Autodesk Inventor part; units mm, degrees
ref_plane "YZ Plane" through (0, 0, 0) normal (1, 0, 0) x (0, 1, 0)
ref_plane "XZ Plane" through (0, 0, 0) normal (0, 1, 0) x (-1, 0, 0)
ref_plane "XY Plane" through (0, 0, 0) normal (0, 0, 1) x (1, 0, 0)
sketch "Sketch1" plane through (0, 0, 0) normal (0, 1, 0) x (-1, 0, 0)
  line L0 (0, 0) -> (464.159, 0) construction
  line L1 (464.159, 0) -> (464.159, -207.7664) construction
  line L2 (464.159, -207.7664) -> (0, -207.7664) construction
  line L3 (0, -207.7664) -> (0, 0) construction
  line L4 (89.199, -168.5726) -> (89.199, -173.9719)
  line L5 (89.199, -173.9719) -> (86.6636, -173.9719)
  line L6 (86.6636, -173.9719) -> (86.6636, -176.4581)
  line L7 (86.6636, -176.4581) -> (71.2328, -176.4581)
  line L8 (71.2328, -176.4581) -> (71.2328, -186.2934)
  line L9 (71.2328, -186.2934) -> (90.3359, -186.2934)
  line L10 (90.3359, -186.2934) -> (90.3359, -179.7626)
  line L11 (90.3359, -179.7626) -> (92.1613, -179.7626)
  line L12 (92.1613, -179.7626) -> (92.1613, -177.2606)
  line L13 (92.1613, -177.2606) -> (99.2738, -177.2606)
  line L14 (99.2738, -177.2606) -> (99.2738, -159.6681)
  line L15 (99.2738, -159.6681) -> (106.4808, -159.6681)
  line L16 (106.4808, -159.6681) -> (106.4808, -177.355)
  line L17 (106.4808, -177.355) -> (116.4572, -177.355)
  line L18 (116.4572, -177.355) -> (116.4572, -149.6917)
  line L19 (116.4572, -149.6917) -> (109.1915, -149.6917)
  line L20 (109.1915, -149.6917) -> (109.1915, -140.7968)
  line L21 (109.1915, -140.7968) -> (99.2738, -140.7968)
  line L22 (99.2738, -140.7968) -> (99.2738, -131.8637)
  line L23 (99.2738, -131.8637) -> (90.1524, -131.8637)
  line L24 (90.1524, -131.8637) -> (90.1524, -126.827)
  line L25 (90.1524, -126.827) -> (92.1613, -126.827)
  line L26 (92.1613, -126.827) -> (92.1613, -124.6793)
  line L27 (92.1613, -124.6793) -> (99.2738, -124.6793)
  line L28 (99.2738, -124.6793) -> (99.2738, -114.8781)
  line L29 (99.2738, -114.8781) -> (89.326, -114.8781)
  line L30 (89.326, -114.8781) -> (89.326, -121.2519)
  line L31 (89.326, -121.2519) -> (86.6636, -121.2519)
  line L32 (86.6636, -121.2519) -> (86.6636, -122.9811)
  line L33 (86.6636, -122.9811) -> (80.2684, -122.9811)
  line L34 (80.2684, -122.9811) -> (80.2684, -131.8637)
  line L35 (67.5567, -131.8637) -> (80.2684, -131.8637)
  line L36 (67.602, -168.5726) -> (89.199, -168.5726)
  line L37 (46.005, -168.6259) -> (46.0183, -174.0251)
  line L38 (46.0183, -174.0251) -> (48.5537, -174.0188)
  line L39 (48.5537, -174.0188) -> (48.5598, -176.5051)
  line L40 (48.5598, -176.5051) -> (63.9906, -176.467)
  line L41 (63.9906, -176.467) -> (64.0148, -186.3023)
  line L42 (64.0148, -186.3023) -> (44.9117, -186.3494)
  line L43 (44.9117, -186.3494) -> (44.8956, -179.8186)
  line L44 (44.8956, -179.8186) -> (43.0703, -179.8231)
  line L45 (43.0703, -179.8231) -> (43.0641, -177.3211)
  line L46 (43.0641, -177.3211) -> (35.9516, -177.3387)
  line L47 (35.9516, -177.3387) -> (35.9083, -159.7462)
  line L48 (35.9083, -159.7462) -> (28.7013, -159.7639)
  line L49 (28.7013, -159.7639) -> (28.7449, -177.4508)
  line L50 (28.7449, -177.4508) -> (18.7685, -177.4754)
  line L51 (18.7685, -177.4754) -> (18.7003, -149.8121)
  line L52 (18.7003, -149.8121) -> (26.8729, -149.792)
  line L53 (26.8729, -149.792) -> (26.8509, -140.8972)
  line L54 (26.8509, -140.8972) -> (35.8617, -140.875)
  line L55 (35.8617, -140.875) -> (35.8397, -131.9419)
  line L56 (35.8397, -131.9419) -> (44.9611, -131.9194)
  line L57 (44.9611, -131.9194) -> (44.9487, -126.8827)
  line L58 (44.9487, -126.8827) -> (42.9398, -126.8877)
  line L59 (42.9398, -126.8877) -> (42.9345, -124.7399)
  line L60 (42.9345, -124.7399) -> (35.822, -124.7574)
  line L61 (35.822, -124.7574) -> (35.7979, -114.9563)
  line L62 (35.7979, -114.9563) -> (45.7457, -114.9318)
  line L63 (45.7457, -114.9318) -> (45.7614, -121.3056)
  line L64 (45.7614, -121.3056) -> (48.4237, -121.299)
  line L65 (48.4237, -121.299) -> (48.428, -123.0282)
  line L66 (48.428, -123.0282) -> (54.8232, -123.0124)
  line L67 (54.8232, -123.0124) -> (54.8451, -131.8951)
  line L68 (67.5567, -131.8637) -> (54.8451, -131.8951)
  line L69 (67.602, -168.5726) -> (46.005, -168.6259)
  line L70 (46.7205, -142.4875) -> (53.9587, -142.4875)
  line L71 (53.9587, -142.4875) -> (53.9587, -149.7258)
  line L72 (53.9587, -149.7258) -> (46.7205, -149.7258)
  line L73 (46.7205, -149.7258) -> (46.7205, -142.4875)
  line L74 (82.0966, -142.4875) -> (89.3348, -142.4875)
  line L75 (89.3348, -142.4875) -> (89.3348, -149.7258)
  line L76 (89.3348, -149.7258) -> (82.0966, -149.7258)
  line L77 (82.0966, -149.7258) -> (82.0966, -142.4875)
  dimension "d30" = 90
  dimension "d32" = 90
  dimension "d34" = 90
  dimension "d35" = 90
  dimension "d36" = 7.2382
  dimension "d39" = 7.2382
  dimension "d40" = 7.2382
  dimension "d41" = 7.2382
  dimension "d43" = 19.8567
  dimension "d44" = 28.1378
extrude "Extrusion1" add sketch "Sketch1" along normal blind 6.35
equation "\"d39\" = d36"
equation "\"d40\" = d36"
properties part number "Monster2"
Verification items for the finished model (mm, model axes). A direction names the side the tool comes from. Give positions to 0.01 mm unless a question says otherwise; leave off trailing zeros. Write each loop counter-clockwise with the first axis right and the second up, starting at its lowest first coordinate (ties: lowest second). Pieces come first, ordered by that corner, then holes. Notation, with made-up numbers: M -36.5,-3.75 L -24.5,-3.75 A27 cw -24.5,34.25 Z; hole C -17.75,40 d7. An arc over 180 degrees is marked long. Use CSV: the item, a comma, the result in double quotes.
1) Cross-section at B-B (z = -146). Enter the section's corners in (x, y).
Final values:
outline,"M -109.19,0 L -89.33,0 L -89.33,6.35 L -109.19,6.35 Z; M -82.1,0 L -53.96,0 L -53.96,6.35 L -82.1,6.35 Z; M -46.72,0 L -26.86,0 L -26.86,6.35 L -46.72,6.35 Z"
2) Cross-section at D-D (y = 2.5). State how many separate pieces and enclosed holes the cut face has, plus the area to 3 significant figures.
Final values:
separate pieces,"1"
enclosed holes,"2"
area,"4,040 mm²"
3) Cross-section at A-A (x = -76.5). Enter the section's corners in (y, z).
Final values:
outline,"M 0,-186.29 L 6.35,-186.29 L 6.35,-176.46 L 0,-176.46 Z; M 0,-168.57 L 6.35,-168.57 L 6.35,-131.86 L 0,-131.86 Z"
4) Go/stop test with flat-tipped pins: pin 1 Ø1.9 at (y, z) = (4, -119) entering from -X; pin 2 Ø1.9 at (x, y) = (-95, 4) entering from -Z; pin 3 Ø2 at (x, y) = (-88, 3) entering from +Z; pin 4 Ø1 at (x, z) = (-93.5, -127.5) entering from +Y. Record where each tip stops, or that it passes through.
Final values:
pin 1,"x = -99.27"
pin 2,"z = -177.26"
pin 3,"z = -121.25"
pin 4,"through"
5) Release check for a two-part mould opening along Z. For faces 5 (the face through (-81, 3, -186.293)), 6 (the face through (-67, 6.35, -150)), 7 (the face through (-86.664, 3, -175)) record: released by +Z, released by -Z, zero draft, split by the parting line, or undercut.
Final values:
face 5,"released by -Z"
face 6,"zero draft"
face 7,"undercut"
6) Material ranges on line 1 along X through (y, z) = (4.5, -175); line 2 along Z through (x, y) = (-86, 1.5); line 3 along X through (y, z) = (5, -171), recorded low to high.
Final values:
line 1,"-116.46 to -106.48, -99.27 to -86.66, -48.56 to -35.95, -28.74 to -18.76"
line 2,"-186.29 to -176.46, -168.57 to -149.73, -142.49 to -122.98"
line 3,"-116.46 to -106.48, -99.27 to -89.2, -46.01 to -35.94, -28.73 to -18.75"
7) Cross-section at C-C (z = -129). Enter the section's corners in (x, y).
Final values:
outline,"M -90.15,0 L -80.27,0 L -80.27,6.35 L -90.15,6.35 Z; M -54.84,0 L -44.95,0 L -44.95,6.35 L -54.84,6.35 Z"
8) Access from +Z, -Z, +X, -X, +Y, -Y to the whole of each face (thin tool, end or side, straight path). Record for faces 1 (the face through (-109.192, 3, -145)), 2 (the face through (-95, 3, -131.864)), 3 (the face through (-103, 3, -159.668)), 4 (the face through (-50, 3, -149.726)).
Final values:
face 1,"+Z, -X, +Y, -Y"
face 2,"-X, +Y, -Y"
face 3,"-Z, +Y, -Y"
face 4,"+Y, -Y"
